from build123d import *

# Parameters (mm, degrees)
F0_W     = 101.3
F0_H     = 91.6
F1_DEPTH = 39.9
F3_DEPTH = 39.9
F4_W     = 91.3
F4_H     = 81.6
F5_DEPTH = 25
F7_DEPTH = 40


with BuildPart() as f1:
    # F0 (on Top) → F1 (new body)
    with BuildSketch(Plane.XY):
        Rectangle(F0_W, F0_H)
    extrude(amount=F1_DEPTH)

    # F2 (on face) → F3 (cut)
    with BuildSketch(Plane.XY.offset(39.9)):
        Polygon((50.65, 45.8), (-38.65, 45.8), (-38.65, 43.8), (-48.65, 43.8), (-48.65, 41.8), (-46.65, 41.8), (-46.65, -41.8), (46.65, -41.8), (46.65, -43.8), (48.65, -43.8), (48.65, -33.8), (50.65, -33.8), align=None)
    extrude(amount=-F3_DEPTH, mode=Mode.SUBTRACT)

    # F4 (on face) → F5 (cut)
    with BuildSketch(Plane(origin=(0, 0, 0), x_dir=(1, 0, 0), z_dir=(0, 0, -1))):
        Rectangle(F4_W, F4_H)
    extrude(amount=-F5_DEPTH, mode=Mode.SUBTRACT)

    # F6 (on face) → F7 (cut)
    with BuildSketch(Plane.XY.offset(39.9)):
        Polygon((-48.65, 39.8), (-50.65, 39.8), (-50.65, -45.8), (44.65, -45.8), (44.65, -43.8), (-48.65, -43.8), align=None)
    extrude(amount=-F7_DEPTH, mode=Mode.SUBTRACT)


solid = f1.part
Read the model definition and answer for the solid it produces. Units are mm, in the model's axes. A direction names the side the tool comes from. Coordinates: 2 decimals unless noted, no trailing zeros. Order: outer loops, then holes, each group sorted by start corner. A loop starts at its lowest first (then second) coordinate and runs counter-clockwise, first axis right, second up. Notation, with made-up numbers: (72.5, -13.75) - (116.5, -13.75) arc R20 cw to (116.5, 18.25) - close; hole circle Ø8 at (-25.75, 49.25). An arc over 180 degrees is marked (long way). Use one line per item in the form item = value.
(1) Section D-D, the plane x = 11 is taken. Give the vertices of the cut face in (y, z).
Computed values:
outline = (-43.8, 0) - (-41.8, 0) - (-41.8, 39.9) - (-43.8, 39.9) - close
(2) Section A-A, the plane x = -42 is taken. Give the vertices of the cut face in (y, z).
Computed values:
outline = (-43.8, 0) - (-41.8, 0) - (-41.8, 39.9) - (-43.8, 39.9) - close; (43.8, 0) - (45.8, 0) - (45.8, 39.9) - (43.8, 39.9) - close
(3) Straight lines are drawn through the part: L1, parallel to Y at x = -40.5, z = 24.5; L2, parallel to Y at x = -33.5, z = 33.5; L3, parallel to X at y = -19.5, z = 12. For each, find the intervals that lie inside material, in ascending order.
Computed values:
L1 = -43.8 to -41.8, 43.8 to 45.8
L2 = -43.8 to -41.8
L3 = -48.65 to -46.65
(4) Section B-B, the plane z = 13 is taken. Give the vertices of the cut face in (x, y).
Computed values:
outline = (-50.65, 39.8) - (-48.65, 39.8) - (-48.65, -43.8) - (44.65, -43.8) - (44.65, -45.8) - (50.65, -45.8) - (50.65, -33.8) - (48.65, -33.8) - (48.65, -43.8) - (46.65, -43.8) - (46.65, -41.8) - (-46.65, -41.8) - (-46.65, 41.8) - (-48.65, 41.8) - (-48.65, 43.8) - (-38.65, 43.8) - (-38.65, 45.8) - (-50.65, 45.8) - close
(5) Section C-C, the plane y = 31 is taken. Give the vertices of the cut face in (x, z), then the cut area to 3 significant figures.
Computed values:
outline = (-48.65, 0) - (-46.65, 0) - (-46.65, 39.9) - (-48.65, 39.9) - close
area = 79.8 mm²
(6) Given pin 1 Ø1 at (x, z) = (49.5, 23.5) entering from +Y; pin 2 Ø0.6 at (y, z) = (-44.5, 13.5) entering from -X; pin 3 Ø11 at (x, z) = (-42, 14.5) entering from -Y, each flat-ended and moving along its own axis, determine where each tip first touches the part or whether it passes through.
Computed values:
pin_1 = -33.8
pin_2 = 44.65
pin_3 = -43.8
(7) Which of the six approach directions +Z, -Z, +X, -X, +Y, -Y give full straight-line access (tool end or side, diameter ignored) to faces 5 (the face through (48, -45.8, 20)), 6 (the face through (-44, 43.8, 20)), 7 (the face through (-1, -43.8, 20))?
Computed values:
face_5 = +Z, -Z, +X, -X, -Y
face_6 = +Z, -Z, +X
face_7 = +Z, -Z, -X, -Y
(8) For a pull along X with two mould halves and no side action, classify faces 1 (the face through (48.65, -39, 20)), 2 (the face through (-1, -41.8, 20)), 3 (the face through (50.65, -40, 20)), 4 (the face through (-50.65, 43, 20)) as pulls with the +X half, pulls with the -X half, needs draft (parallel to the pull), parting line crosses it, or undercut.
Computed values:
face_1 = undercut
face_2 = undercut
face_3 = pulls with the +X half
face_4 = pulls with the -X half
